```python
from build123d import *

# Parameters (mm, degrees)
BOX001_W      = 10
BOX001_H      = 6
BOX001_DEPTH  = 1
CHAMFER_SIZE  = 0.9
ARRAY_X_COUNT = 5
ARRAY_X_PITCH = 11
ARRAY_Y_COUNT = 4
ARRAY_Y_PITCH = 7
BOX_W         = 54
BOX_H         = 27
BOX_DEPTH     = 1


with BuildPart() as array:
    # Box001 → Box001 (new body)
    with BuildSketch(Plane.XY.offset(1)):
        with Locations((5, 3)):
            Rectangle(BOX001_W, BOX001_H)
    extrude(amount=BOX001_DEPTH)

    # Chamfer
    chamfer_edges = [array.edges().sort_by_distance(p)[0] for p in [
        (0, 3, 2),
        (10, 3, 2),
        (5, 0, 2),
        (5, 6, 2),
    ]]
    chamfer(chamfer_edges, length=CHAMFER_SIZE)

    # Array X: Array ×5


with BuildPart() as array_1:
    add(array.part)
    with Locations(*[(i * ARRAY_X_PITCH, 0, 0) for i in range(1, ARRAY_X_COUNT)]):
        add(array.part)

    # Array Y: Array ×4


with BuildPart() as array_2:
    add(array_1.part)
    with Locations(*[(0, i * ARRAY_Y_PITCH, 0) for i in range(1, ARRAY_Y_COUNT)]):
        add(array_1.part)


with BuildPart() as fusion:
    # Box → Box (new body)
    with BuildSketch(Plane.XY):
        with Locations((27, 13.5)):
            Rectangle(BOX_W, BOX_H)
    extrude(amount=BOX_DEPTH)

    # Fusion: union Array
    add(array_2.part)


solid = fusion.part
```
CAD build for the part. Positions are in the model's coordinates, mm. Round coordinates to 2 decimals unless told otherwise and drop trailing zeros. Order: outer loops, then holes, each group sorted by start corner. A loop starts at its lowest first (then second) coordinate and runs counter-clockwise, first axis right, second up.
Item 1: Saw through at C-C on x = 45.5. Write the cut outline in (y, z), then the cut area to 3 significant figures.
Item 2: Pin check, flat tips, straight feed: pin 1 (2 mm diameter, centred on x = 20.5, y = 20.5, fed in from +Z); pin 2 (1.5 mm diameter, centred on x = 14.5, y = 7, fed in from +Z); pin 3 (5 mm diameter, centred on x = 33.5, y = 19.5, fed in from -Z); pin 4 (1 mm diameter, centred on y = 21.5, z = 2, fed in from -X). Stop position of each tip, or through.
Item 3: Mould opens along Y. For faces 1 (the face through (27, 17, 2)), 2 (the face through (24.9, 13.6, 1)) say: pulls with the +Y half, pulls with the -Y half, needs draft (parallel to the pull), parting line crosses it, or undercut.
Item 4: Probe line 1 along Y through (x, z) = (29, 1.1); line 2 along X through (y, z) = (18, 1.05); line 3 along Y through (x, z) = (12.5, 1.3). List the from-to ranges inside material, lowest first.
Item 5: Saw through at B-B on z = 1.6. State how many separate pieces and enclosed holes the cut face has, then the cut area to 3 significant figures.
Reported:
1. outline: (0, 0) - (27, 0) - (27, 1.1) - (26.1, 2) - (21.9, 2) - (21, 1.1) - (21, 1) - (20, 1) - (20, 1.1) - (19.1, 2) - (14.9, 2) - (14, 1.1) - (14, 1) - (13, 1) - (13, 1.1) - (12.1, 2) - (7.9, 2) - (7, 1.1) - (7, 1) - (6, 1) - (6, 1.1) - (5.1, 2) - (0.9, 2) - (0, 1.1) - close
1. area: 47.8 mm2
2. pin 1: stops at z = 1.6
2. pin 2: stops at z = 1.85
2. pin 3: stops at z = 0
2. pin 4: stops at x = 0.4
3. face 1: needs draft
3. face 2: undercut
4. line 1: y = 0 to 6, 7 to 13, 14 to 20, 21 to 27
4. line 2: x = 0 to 10, 11 to 21, 22 to 32, 33 to 43, 44 to 54
4. line 3: y = 0.2 to 5.8, 7.2 to 12.8, 14.2 to 19.8, 21.2 to 26.8
5. separate pieces: 20
5. enclosed holes: 0
5. area: 900 mm2
